```python
from build123d import *

# Parameters (mm, degrees)
SKETCH_W        = 37.5
SKETCH_H        = 39
PAD_DEPTH       = 2.5
SKETCH001_R     = 10.75
POCKET_DEPTH    = 5
SKETCH002_R     = 1.75
SKETCH002_W     = 2
SKETCH002_H     = 3.5
SKETCH002_W_2   = 3.5
SKETCH002_H_2   = 2
SKETCH002_W_3   = 11
SKETCH002_H_3   = 4.5
POCKET001_DEPTH = 5
FILLET_R        = 4
SKETCH003_R     = 1.6
POCKET002_DEPTH = 1.1
SKETCH004_R     = 0.9
POCKET003_DEPTH = 5
CHAMFER_SIZE    = 1


with BuildPart() as part:
    # Sketch → Pad (new body)
    with BuildSketch(Plane.XY):
        Rectangle(SKETCH_W, SKETCH_H)
    extrude(amount=PAD_DEPTH)

    # Sketch001 (on Face6 of Pad) → Pocket (cut)
    with BuildSketch(Plane.XY.offset(2.5)):
        Circle(SKETCH001_R)
    extrude(amount=-POCKET_DEPTH, mode=Mode.SUBTRACT)

    # Sketch002 (on Face5 of Pocket) → Pocket001 (cut)
    with BuildSketch(Plane.XY.offset(2.5)):
        with Locations((-9, 12)):
            Circle(SKETCH002_R)
        with Locations((9, -12)):
            Circle(SKETCH002_R)
        with Locations((11.606602, 0)):
            Rectangle(SKETCH002_W, SKETCH002_H)
        with Locations((-11.606602, 0)):
            Rectangle(SKETCH002_W, SKETCH002_H)
        with Locations((0, 11.606602)):
            Rectangle(SKETCH002_W_2, SKETCH002_H_2)
        with Locations((0, -11.486477)):
            Rectangle(SKETCH002_W_3, SKETCH002_H_3)
    extrude(amount=-POCKET001_DEPTH, mode=Mode.SUBTRACT)

    # Fillet
    fillet_edges = [part.edges().sort_by_distance(p)[0] for p in [
        (18.75, -19.5, 1.25),
        (-18.75, -19.5, 1.25),
        (18.75, 19.5, 1.25),
        (-18.75, 19.5, 1.25),
    ]]
    fillet(fillet_edges, radius=FILLET_R)

    # Sketch003 (on Face5 of Fillet) → Pocket002 (cut)
    with BuildSketch(Plane.XY.offset(2.5)):
        with Locations((-15, 0)):
            Circle(SKETCH003_R)
        with Locations((15, 0)):
            Circle(SKETCH003_R)
    extrude(amount=-POCKET002_DEPTH, mode=Mode.SUBTRACT)

    # Sketch004 (on Face31 of Pocket002) → Pocket003 (cut)
    with BuildSketch(Plane.XY.offset(1.4)):
        with Locations((-15, 0)):
            Circle(SKETCH004_R)
        with Locations((15, 0)):
            Circle(SKETCH004_R)
    extrude(amount=-POCKET003_DEPTH, mode=Mode.SUBTRACT)

    # Chamfer
    chamfer_edges = [part.edges().sort_by_distance(p)[0] for p in [
        (-18.75, 0, 2.5),
    ]]
    chamfer(chamfer_edges, length=CHAMFER_SIZE)


solid = part.part
```
Could you check a few things on this model? Use its own coordinates, in mm. A direction names the side the tool comes from. Give positions to 0.01 mm unless a question says otherwise; leave off trailing zeros. Order: outer loops, then holes, each group sorted by start corner. A loop starts at its lowest first (then second) coordinate and runs counter-clockwise, first axis right, second up.
Q1. We'd pull the mould along X, two halves only. Please class faces 1 (the cylindrical face through (9.9, -10.5, 1.3)), 2 (the conical face through (17.088, -17.787, 2.229)), 3 (the flat face through (0, -19.5, 1)): +X half, -X half, draft (parallel to the pull), parting line (faces both ways), or undercut.
Q2. I'm going to push a flat-ended pin straight in: P1, Ø3, axis at x = 15, y = 0, coming from the +Z side. Where does the tip first touch, or does it pass through?
Q3. Suppose I cut it at C-C, the plane z = 0.4. Write out the boundary of the cut face in (x, y), and give its area (3 significant figures).
Q4. If I drill on line 1 along X through (y, z) = (-10, 1.25); line 2 along Y through (x, z) = (15, 0.85); line 3 along Y through (x, z) = (1.5, 0.75), over which ranges is the centre line in solid material (lowest first)?
Q5. Suppose I cut it at D-D, the plane y = 0. Write out the boundary of the cut face in (x, z), and give its area (3 significant figures).
Q6. Suppose I cut it at A-A, the plane y = -12. Write out the boundary of the cut face in (x, z).
Q7. Suppose I cut it at B-B, the plane x = 11.5. Write out the boundary of the cut face in (y, z), and give its area (4 significant figures).
Q8. For faces 4 (the flat face through (-18.24, -0.22, 2.01)), 5 (the cylindrical face through (8.844, -6.112, 1.268)), 6 (the flat face through (-14, -1, 1.4)), which set-ups out of +Z, -Z, +X, -X, +Y, -Y let a thin tool reach every point of the face, with its end or its side?
Solution:
1. face 1: undercut
1. face 2: +X half
1. face 3: draft
2. P1: stops at z = 1.4
3. outline: (-18.75, -15.5) arc R4 ccw to (-14.75, -19.5) - (14.75, -19.5) arc R4 ccw to (18.75, -15.5) - (18.75, 15.5) arc R4 ccw to (14.75, 19.5) - (-14.75, 19.5) arc R4 ccw to (-18.75, 15.5) - close; hole circle Ø1.8 at (-15, 0); hole (-12.61, -1.75) - (-10.61, -1.75) arc R10.75 ccw to (-5.5, -9.24) - (-5.5, -13.74) - (5.5, -13.74) - (5.5, -9.24) arc R10.75 ccw to (10.61, -1.75) - (12.61, -1.75) - (12.61, 1.75) - (10.61, 1.75) arc R10.75 ccw to (1.75, 10.61) - (1.75, 12.61) - (-1.75, 12.61) - (-1.75, 10.61) arc R10.75 ccw to (-10.61, 1.75) - (-12.61, 1.75) - close; hole circle Ø3.5 at (-9, 12); hole circle Ø3.5 at (9, -12); hole circle Ø1.8 at (15, 0)
3. area: 1,000 mm2
4. line 1: x = -18.75 to -5.5, 5.5 to 18.75
4. line 2: y = -19.49 to -0.9, 0.9 to 19.49
4. line 3: y = -19.5 to -13.74, 12.61 to 19.5
5. outline: (-18.75, 0) - (-15.9, 0) - (-15.9, 1.4) - (-16.6, 1.4) - (-16.6, 2.5) - (-17.75, 2.5) - (-18.75, 1.5) - close; (-14.1, 0) - (-12.61, 0) - (-12.61, 2.5) - (-13.4, 2.5) - (-13.4, 1.4) - (-14.1, 1.4) - close; (12.61, 0) - (14.1, 0) - (14.1, 1.4) - (13.4, 1.4) - (13.4, 2.5) - (12.61, 2.5) - close; (15.9, 0) - (18.75, 0) - (18.75, 1.5) - (17.75, 2.5) - (16.6, 2.5) - (16.6, 1.4) - (15.9, 1.4) - close
5. area: 17.6 mm2
6. outline: (-18.75, 0) - (-5.5, 0) - (-5.5, 2.5) - (-17.75, 2.5) - (-18.75, 1.5) - close; (5.5, 0) - (7.25, 0) - (7.25, 2.5) - (5.5, 2.5) - close; (10.75, 0) - (18.75, 0) - (18.75, 1.5) - (17.75, 2.5) - (10.75, 2.5) - close
7. outline: (-19.5, 0) - (-1.75, 0) - (-1.75, 2.5) - (-18.5, 2.5) - (-19.5, 1.5) - close; (1.75, 0) - (19.5, 0) - (19.5, 1.5) - (18.5, 2.5) - (1.75, 2.5) - close
7. area: 87.75 mm2
8. face 4: +Z, -X, +Y, -Y
8. face 5: +Z, -Z
8. face 6: +Z
